Print and shaded views of the part. All mm, measured from the part's lowest x, y and z. A direction names the side the tool comes from. Round coordinates to 2 decimals unless told otherwise and drop trailing zeros. Write each loop counter-clockwise with the first axis right and the second up, starting at its lowest first coordinate (ties: lowest second). Pieces come first, ordered by that corner, then holes. Notation, with made-up numbers: (73, -12) - (99, -12) arc R17 ccw to (99, 4) - close; hole circle Ø1 at (23, 62). An arc over 180 degrees is marked (long way). Put each result on its own line as item: value. Start each with the question number.
Item 1: Mould opens along X. For the marked faces 3, 4 and 5 say: released by +X, released by -X, zero draft, split by the parting line, or undercut.
Item 2: Cut at A-A (y = 80). Give the cut face in (x, z), and give its area (3 significant figures).
Item 3: Drill centre lines: line 1 (Y direction, x = 50, z = 83); line 2 (Y direction, x = 50, z = 8); line 3 (Y direction, x = 47, z = 39.5). Where is each one in solid material? Low to high. Write a range as from..to.
Item 4: 3-axis set-ups, long thin cutter, end or side, ignore diameter. For the marked faces 1 and 2: which of +Z, -Z, +X, -X, +Y, -Y reach the whole face in a straight line?
Item 5: Cut at C-C (z = 89.5). Give the cut face in (x, y), and give its area (3 significant figures).
Item 6: Pin check, flat tips, straight feed: pin 1 Ø1.5 at (y, z) = (76.5, 44.5) entering from +X; pin 2 Ø1.5 at (y, z) = (45.5, 63.5) entering from -X; pin 3 Ø10 at (x, z) = (66, 58.5) entering from +Y (1 decimal). Stop position of each tip, or through.
Item 7: Cut at D-D (y = 61.5). Give the cut face in (x, z), and give its area (3 significant figures).
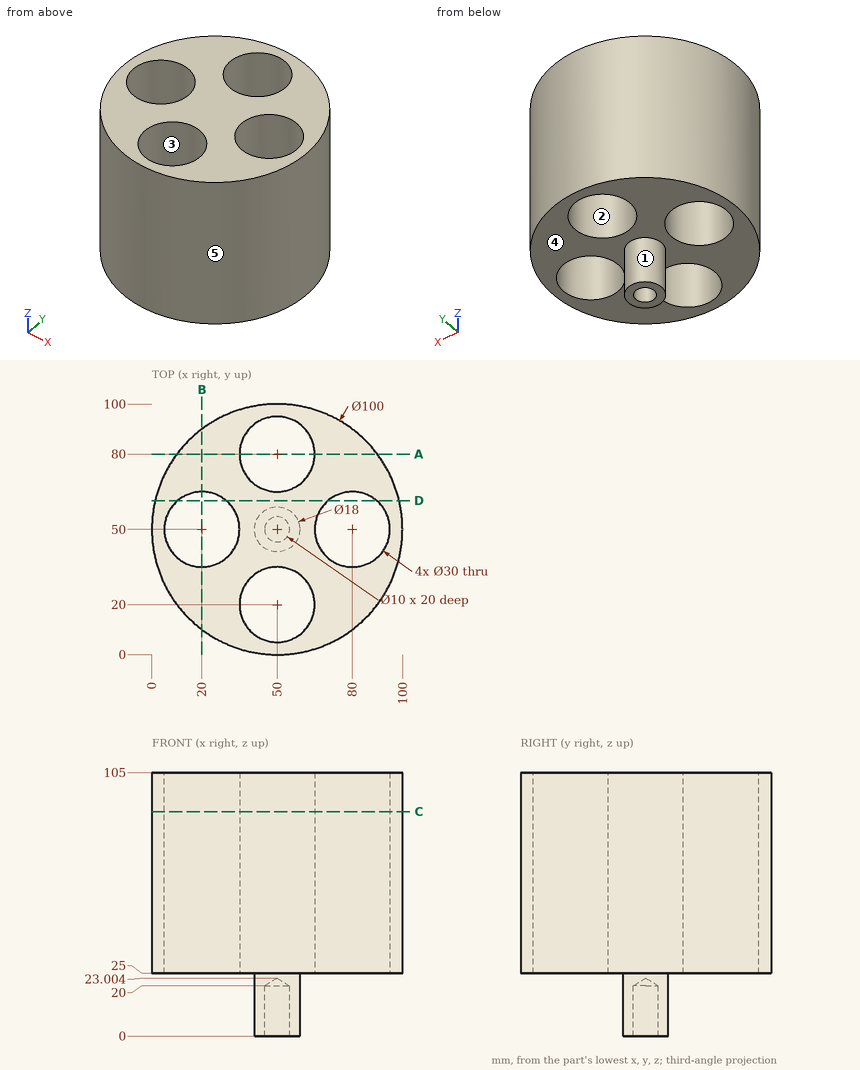
Output values:
1. face 3: undercut
1. face 4: zero draft
1. face 5: split by the parting line
2. outline: (10, 25) - (35, 25) - (35, 105) - (10, 105) - close; (65, 25) - (90, 25) - (90, 105) - (65, 105) - close
2. area: 4,000 mm2
3. line 1: 0..5, 35..65, 95..100
3. line 2: 41..45, 55..59
3. line 3: 0.09..5.3, 34.7..65.3, 94.7..99.91
4. face 1: -Z
4. face 2: +Z, -Z
5. outline: circle Ø100 at (50, 50); hole circle Ø30 at (20, 50); hole circle Ø30 at (50, 20); hole circle Ø30 at (50, 80); hole circle Ø30 at (80, 50)
5. area: 5,030 mm2
6. pin 1: x = 92.86
6. pin 2: x = 0.14
6. pin 3: y = 98.8
7. outline: (1.34, 25) - (10.37, 25) - (10.37, 105) - (1.34, 105) - close; (29.63, 25) - (70.37, 25) - (70.37, 105) - (29.63, 105) - close; (89.63, 25) - (98.66, 25) - (98.66, 105) - (89.63, 105) - close
7. area: 4,700 mm2
